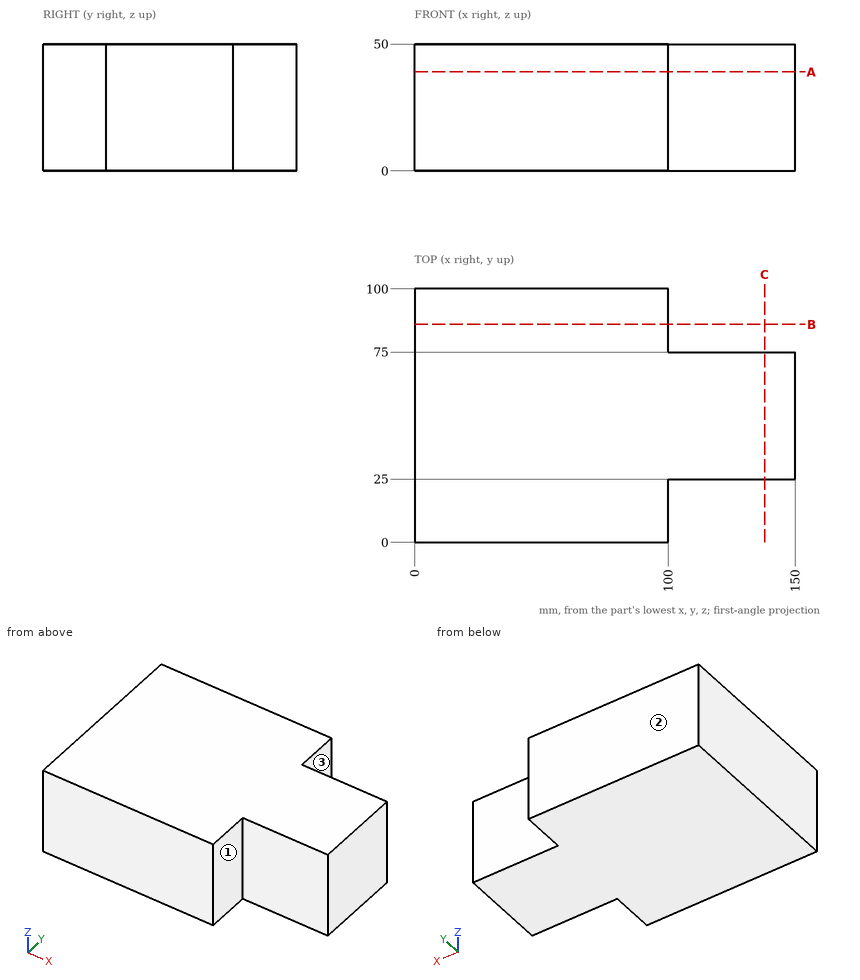
Here's the drawing with two shaded views (mm, measured from the low corner). I have some questions. A direction names the side the tool comes from. Give positions to 0.01 mm unless a question says otherwise; leave off trailing zeros. Order: outer loops, then holes, each group sorted by start corner. A loop starts at its lowest first (then second) coordinate and runs counter-clockwise, first axis right, second up. Notation, with made-up numbers: (0.25, -25) - (26.25, -25) arc R25 cw to (26.25, 10) - close; hole circle Ø5 at (52.25, 7). An arc over 180 degrees is marked (long way). Use a Markdown table: item, result. Add a question column.
Q1. If we section it at B-B on y = 86: Write out the boundary of the cut face in (x, z), plus the area to 3 significant figures.
Q2. On a 3-axis mill with a long thin cutter (end or side, diameter ignored), from which of +Z, -Z, +X, -X, +Y, -Y can I reach the whole of each face in a straight line? I mean the marked faces 1, 2 and 3. Say none if no direction works.
Q3. I'm going to push flat-ended pins straight in: pin 1 (1 mm diameter, centred on x = 82.5, y = 65, fed in from -Z); pin 2 (7.5 mm diameter, centred on y = 81.5, z = 14, fed in from +X); pin 3 (6 mm diameter, centred on x = 118, z = 34, fed in from -Y); pin 4 (15 mm diameter, centred on x = 118.5, z = 13.5, fed in from +Y). Where does each tip first touch, or does it pass through?
Q4. If we section it at A-A on z = 39: Write out the boundary of the cut face in (x, y), plus the area to 3 significant figures.
Q5. Please list where these lines run through material, in increasing order: line 1 along X through (y, z) = (91, 30); line 2 along Y through (x, z) = (138, 48).
Q6. If we section it at C-C on x = 138: Write out the boundary of the cut face in (y, z), plus the area to 3 significant figures.
Answers follow:
| question | item | result |
|---|---|---|
| 1 | outline | (0, 0) - (100, 0) - (100, 50) - (0, 50) - close |
| 1 | area | 5,000 mm^2 |
| 2 | face 1 | +Z, -Z, +X, -Y |
| 2 | face 2 | +Z, -Z, +X, -X, +Y |
| 2 | face 3 | +Z, -Z, +X, +Y |
| 3 | pin 1 | stops at z = 0 |
| 3 | pin 2 | stops at x = 100 |
| 3 | pin 3 | stops at y = 25 |
| 3 | pin 4 | stops at y = 75 |
| 4 | outline | (0, 0) - (100, 0) - (100, 25) - (150, 25) - (150, 75) - (100, 75) - (100, 100) - (0, 100) - close |
| 4 | area | 12,500 mm^2 |
| 5 | line 1 | x = 0 to 100 |
| 5 | line 2 | y = 25 to 75 |
| 6 | outline | (25, 0) - (75, 0) - (75, 50) - (25, 50) - close |
| 6 | area | 2,500 mm^2 |
